Can you work these out from the model? Positions are in its coordinate system, mm. Give positions to 0.01 mm unless a question says otherwise; leave off trailing zeros. Order: outer loops, then holes, each group sorted by start corner. A loop starts at its lowest first (then second) coordinate and runs counter-clockwise, first axis right, second up. Notation, with made-up numbers: (59, 3.5) -> (63, 3.5) arc R19 cw to (63, 32.5) -> close; hole circle Ø2 at (0, 25.5). An arc over 180 degrees is marked (long way). Answer as CSV lines item,"result".
```python
from build123d import *

# Parameters (mm, degrees)
SKETCH_1_R               = 250
EXTRUDE_1_DEPTH          = 20
SKETCH_2_R               = 5
EXTRUDE_2_DEPTH          = 400
SKETCH_3_R               = 15
EXTRUDE_3_DEPTH          = 5
SKETCH_4_R               = 1.65
CUT_EXTRUDE_1_DEPTH      = 5
PATTERN_CIRCULAR_1_COUNT = 4


with BuildPart() as part:
    # 草图1 → 凸台-拉伸1 (new body)
    with BuildSketch(Plane(origin=(0, 0, 0), x_dir=(1, 0, 0), z_dir=(0, 1, 0))):
        with Locations(Location((0, 0, 0), (0, 0, 270))):
            Circle(SKETCH_1_R)
    extrude(amount=EXTRUDE_1_DEPTH)

    # 草图2 → 凸台-拉伸2 (add)
    with BuildSketch(Plane(origin=(0, 20, 0), x_dir=(1, 0, 0), z_dir=(0, 1, 0))):
        with Locations(Location((0, 0, 0), (0, 0, 270))):
            Circle(SKETCH_2_R)
    extrude(amount=EXTRUDE_2_DEPTH)

    # 草图3 → 凸台-拉伸3 (add)
    with BuildSketch(Plane(origin=(0, 420, 0), x_dir=(1, 0, 0), z_dir=(0, 1, 0))):
        with Locations(Location((0, 0, 0), (0, 0, 270))):
            Circle(SKETCH_3_R)
    extrude(amount=EXTRUDE_3_DEPTH)

    # 草图4 → 切除-拉伸1 (cut)
    with BuildSketch(Plane(origin=(0, 425, 0), x_dir=(1, 0, 0), z_dir=(0, 1, 0))):
        with Locations(Location((-7, 0, 0), (0, 0, 270))):
            Circle(SKETCH_4_R)
    cut_extrude_1 = extrude(amount=-CUT_EXTRUDE_1_DEPTH, mode=Mode.SUBTRACT)

    # 阵列(圆周)1: 切除-拉伸1 ×4 about axis
    pattern_circular_1_axis = Axis((0, 0, 0), (0, 1, 0))
    for i in range(1, PATTERN_CIRCULAR_1_COUNT):
        add(cut_extrude_1.rotate(pattern_circular_1_axis, i * 360 / PATTERN_CIRCULAR_1_COUNT), mode=Mode.SUBTRACT)


solid = part.part
```
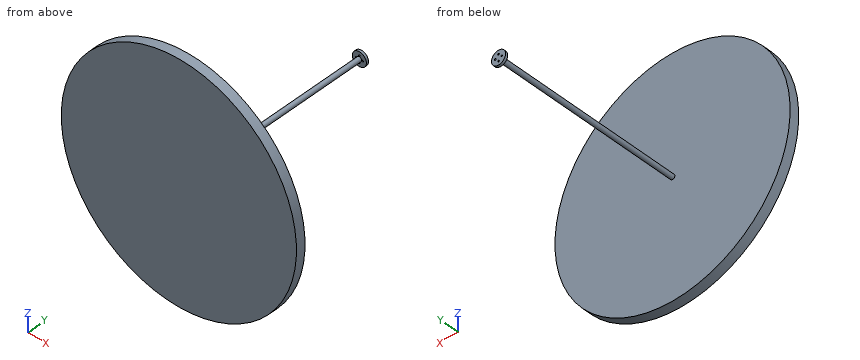
Item 1: For pin 1 (2 mm diameter, centred on x = 7, z = 0, fed in from +Y), with a flat end and sliding along its axis, tell me the tip position at first contact or that it passes through.
Numbers:
pin 1,"stops at y = 20"
Item 2: Imagine slicing it at B-B, the plane x = 196. Please give me the cut outline in (y, z), then the cut area to 3 significant figures.
Numbers:
outline,"(0, -155.19) -> (20, -155.19) -> (20, 155.19) -> (0, 155.19) -> close"
area,"6,210 mm²"
Item 3: Please list where these lines run through material, in increasing order: line 1 along X through (y, z) = (422.25, 0); line 2 along Y through (x, z) = (-13.5, -4); line 3 along Y through (x, z) = (-17, -96).
Numbers:
line 1,"x = -15 to -8.65, -5.35 to 5.35, 8.65 to 15"
line 2,"y = 0 to 20, 420 to 425"
line 3,"y = 0 to 20"
Item 4: Imagine slicing it at C-C, the plane z = 127.5. Please give me the cut outline in (x, y), then the cut area to 3 significant figures.
Numbers:
outline,"(-215.04, 0) -> (215.04, 0) -> (215.04, 20) -> (-215.04, 20) -> close"
area,"8,600 mm²"
Item 5: Imagine slicing it at A-A, the plane y = 140. Please give me the cut outline in (x, z), then the cut area to 3 significant figures.
Numbers:
outline,"circle Ø10 at (0, 0)"
area,"78.5 mm²"
